```python
from build123d import *

# Parameters (mm, degrees)
F0_W     = 127.508
F0_H     = 13.716
F1_DEPTH = 2.54
F2_R     = 5.08
F3_DEPTH = 127


with BuildPart() as f1:
    # F0 (on Top) → F1 (new body)
    with BuildSketch(Plane.XY):
        Rectangle(F0_W, F0_H)
    extrude(amount=F1_DEPTH)

    # F2 (on Top) → F3 (join)
    with BuildSketch(Plane.XY):
        Circle(F2_R)
        with Locations((19.05, 0)):
            Circle(F2_R)
        with Locations((38.1, 0)):
            Circle(F2_R)
        with Locations((57.15, 0)):
            Circle(F2_R)
        with Locations((-19.05, 0)):
            Circle(F2_R)
        with Locations((-38.1, 0)):
            Circle(F2_R)
        with Locations((-57.15, 0)):
            Circle(F2_R)
    extrude(amount=F3_DEPTH)


solid = f1.part
```
Model file for the job. Use its own axes, mm. A direction names the side the tool comes from. Round coordinates to 2 decimals unless told otherwise and drop trailing zeros. Loops run counter-clockwise (first coordinate to the right, second up) from the corner with the lowest first, then second, coordinate; pieces in that order, holes last. Notation, with made-up numbers: M 67.25,55.25 L 75.25,55.25 A27 cw 75.25,75.25 Z; hole C 58.5,57.5 d2. An arc over 180 degrees is marked long. Put each result on its own line as item: value. Start each with the question number.
Item 1: Cut at D-D (x = -49). List the corners of the cut face in (y, z), then the cut area to 3 significant figures.
Item 2: Drop flat-ended pins along their axis: P1, Ø3, axis at y = 1, z = 14, coming from the -X side; P2, Ø6, axis at y = 3.5, z = 21, coming from the +X side; P3, Ø8, axis at x = 50, z = 45.5, coming from the +Y side. Give the stop position or say it passes through.
Item 3: 3-axis set-ups, long thin cutter, end or side, ignore diameter. For faces 1 (the face through (-1, 0, 0)), 2 (the face through (52.075, 0.223, 63.899)): which of +Z, -Z, +X, -X, +Y, -Y reach the whole face in a straight line?
Item 4: Drill centre lines: line 1 along Z through (x, y) = (29, -2.5); line 2 along Y through (x, z) = (41, 57); line 3 along Y through (x, z) = (-37, 116). Where is each one in solid material? Low to high.
Item 5: Cut at B-B (x = 57.15). List the corners of the cut face in (y, z), then the cut area to 3 significant figures.
Item 6: Cut at A-A (z = 28.5). List the corners of the cut face in (x, y), then the cut area to 3 significant figures.
Item 7: Mould opens along X. For faces 3 (the face through (-1, -6, 2.54)), 4 (the face through (-57, 0, 127)) say: released by +X, released by -X, zero draft, split by the parting line, or undercut.
Answer block:
1. outline: M -6.86,0 L 6.86,0 L 6.86,2.54 L -6.86,2.54 Z
1. area: 34.8 mm2
2. P1: x = -62.23
2. P2: x = 62.21
2. P3: y = 3.99
3. face 1: -Z, +X, -X, +Y, -Y
3. face 2: +Z
4. line 1: 0 to 2.54
4. line 2: -4.17 to 4.17
4. line 3: -4.96 to 4.96
5. outline: M -6.86,0 L 6.86,0 L 6.86,2.54 L 5.08,2.54 L 5.08,127 L -5.08,127 L -5.08,2.54 L -6.86,2.54 Z
5. area: 1,300 mm2
6. outline: C -57.15,0 d10.16; C -38.1,0 d10.16; C -19.05,0 d10.16; C 0,0 d10.16; C 19.05,0 d10.16; C 38.1,0 d10.16; C 57.15,0 d10.16
6. area: 568 mm2
7. face 3: undercut
7. face 4: zero draft
